Design review of the part built by this model. Coordinates are the model's own, in mm. Coordinates: 2 decimals unless noted, no trailing zeros. Loops run counter-clockwise (first coordinate to the right, second up) from the corner with the lowest first, then second, coordinate; pieces in that order, holes last. Notation, with made-up numbers: (-12.5, -18.5) -> (41.5, -18.5) arc R30 ccw to (41.5, 8.5) -> close; hole circle Ø6 at (-37.5, -38). An arc over 180 degrees is marked (long way). Answer in a Markdown table with one row per item.
Solid Edge part; units mm, degrees
sketch "Sketch1" plane through (0, 0, 0) normal (0, 0, 1) x (1, 0, 0)
  line L0 (-23.094, 40) -> (-46.188, 0)
  line L1 (-46.188, 0) -> (-23.094, -40)
  line L2 (-23.094, -40) -> (23.094, -40)
  line L3 (23.094, -40) -> (46.188, 0)
  line L4 (46.188, 0) -> (23.094, 40)
  line L5 (23.094, 40) -> (-23.094, 40)
extrude "Protrusion1" add sketch "Sketch1" along normal blind 25
hole "Hole_5" at (0, 0, 25) direction (0, 0, -1) diameter 40 end up to next
sketch "Sketch2" plane through (0, 0, 0) normal (0, -1, 0) x (1, 0, 0)
  line L0 (-39.998, 25) -> (-46.188, 25)
  line L1 (-46.188, 25) -> (-46.188, 19.955)
  line L2 (-46.188, 19.955) -> (-39.998, 25)
revolve "RevolvedCutout1" cut sketch "Sketch2" angle 360 about axis through (0, 0, 0) along (0, 0, 1)
(1) Take a section at C-C on z = 22. Give the boundary of the cut face in (x, y), and give its area (3 significant figures).
Evaluation:
| item | result |
|---|---|
| outline | (-43.41, -4.81) -> (-25.87, -35.19) arc R43.68 ccw to (-17.55, -40) -> (17.55, -40) arc R43.68 ccw to (25.87, -35.19) -> (43.41, -4.81) arc R43.68 ccw to (43.41, 4.81) -> (25.87, 35.19) arc R43.68 ccw to (17.55, 40) -> (-17.55, 40) arc R43.68 ccw to (-25.87, 35.19) -> (-43.41, 4.81) arc R43.68 ccw to start; hole circle Ø40 at (0, 0) |
| area | 4,220 mm² |
(2) Take a section at B-B on z = 10.75. Give the boundary of the cut face in (x, y), and give its area (3 significant figures).
Evaluation:
| item | result |
|---|---|
| outline | (-46.19, 0) -> (-23.09, -40) -> (23.09, -40) -> (46.19, 0) -> (23.09, 40) -> (-23.09, 40) -> close; hole circle Ø40 at (0, 0) |
| area | 4,290 mm² |
(3) Draft analysis for pull direction Y (two halves, no side actions). For faces 1 (the flat face through (0, 40, 12)), 2 (the flat face through (34.48, -20.28, 12.32)), 3 (the cylindrical face through (-19.524, 4.336, 12.675)), state which applies: pulls with the +Y half, pulls with the -Y half, needs draft (parallel to the pull), parting line crosses it, or undercut.
Evaluation:
| item | result |
|---|---|
| face 1 | pulls with the +Y half |
| face 2 | pulls with the -Y half |
| face 3 | undercut |
(4) For pin 1 (1.5 mm diameter, centred on x = -25, z = 8.5, fed in from +Y); pin 2 (2 mm diameter, centred on x = 24.5, z = 3, fed in from -Y); pin 3 (2 mm diameter, centred on x = -23.5, z = 5.5, fed in from -Y); pin 4 (1.5 mm diameter, centred on y = 3, z = 7, fed in from -X), all flat-tipped, find the tip position at first contact; note any pin that passes through.
Evaluation:
| item | result |
|---|---|
| pin 1 | stops at y = 38 |
| pin 2 | stops at y = -39.3 |
| pin 3 | stops at y = -40 |
| pin 4 | stops at x = -44.89 |
(5) To check wall thickness, follow probe 1 along X at (y, z) = (0, 16.75); probe 2 along Y at (x, z) = (0, 12.25); probe 3 along X at (y, z) = (-16, 16.5). State the ranges of each line that lie inside material, in increasing order.
Evaluation:
| item | result |
|---|---|
| probe 1 | x = -46.19 to -20, 20 to 46.19 |
| probe 2 | y = -40 to -20, 20 to 40 |
| probe 3 | x = -36.95 to -12, 12 to 36.95 |
